For this review, take the finished solid that the model builds, in its own axes (mm). Coordinates: 2 decimals unless noted, no trailing zeros. Write each loop counter-clockwise with the first axis right and the second up, starting at its lowest first coordinate (ties: lowest second). Pieces come first, ordered by that corner, then holes.
```python
from build123d import *

# Parameters (mm, degrees)
SKETCH1_R               = 3.5
SKETCH1_R_2             = 1.05
BOSS_EXTRUDE1_DEPTH     = 60
CUT_EXTRUDE1_DEPTH      = 0.9
CUT_EXTRUDE1_DEPTH_BACK = 0.9
CUT_EXTRUDE1_START      = -30
SKETCH3_R               = 3.05
CUT_EXTRUDE2_DEPTH      = 0.9
CUT_EXTRUDE2_DEPTH_BACK = 0.9
CUT_EXTRUDE2_START      = -30
SKETCH5_W               = 7
SKETCH5_H               = 7
SKETCH5_R               = 1.05
BOSS_EXTRUDE2_DEPTH     = 60
CUT_EXTRUDE3_DEPTH      = 0.9
CUT_EXTRUDE3_DEPTH_BACK = 0.9
CUT_EXTRUDE3_START      = -30
SKETCH6_R               = 3.05
CUT_EXTRUDE4_DEPTH      = 0.9
CUT_EXTRUDE4_DEPTH_BACK = 0.9
CUT_EXTRUDE4_START      = -30
SKETCH7_W               = 8.533306348
SKETCH7_H               = 4.274424856


with BuildPart() as part:
    # Sketch1 → Boss-Extrude1 (new body)
    with BuildSketch(Plane(origin=(0, 0, 0), x_dir=(1, 0, 0), z_dir=(0, 1, 0))):
        with Locations(Location((0, 0, 0), (0, 0, 270))):
            Circle(SKETCH1_R)
        with Locations(Location((0, 0, 0), (0, 0, 270))):
            Circle(SKETCH1_R_2, mode=Mode.SUBTRACT)
    extrude(amount=BOSS_EXTRUDE1_DEPTH)

    # Sketch3 → Cut-Extrude1 (cut, two sides: drawn at the far end of the back side and taken through both)
    with BuildSketch(Plane(origin=(0, 60, 0), x_dir=(1, 0, 0), z_dir=(0, 1, 0)).offset(CUT_EXTRUDE1_START - CUT_EXTRUDE1_DEPTH_BACK)):
        with Locations(Location((0, 0, 0), (0, 0, 270))):
            Circle(SKETCH3_R)
    extrude(amount=CUT_EXTRUDE1_DEPTH + CUT_EXTRUDE1_DEPTH_BACK, mode=Mode.SUBTRACT)

    # Sketch4 → Cut-Extrude2 (cut, two sides: drawn at the far end of the back side and taken through both)
    with BuildSketch(Plane(origin=(0, 60, 0), x_dir=(1, 0, 0), z_dir=(0, 1, 0)).offset(CUT_EXTRUDE2_START - CUT_EXTRUDE2_DEPTH_BACK)):
        with BuildLine():
            Line((-4.266653174, 0), (4.266653174, 0))
            ThreePointArc((4.266653174, 0), (0, 4.266653174), (-4.266653174, 0))
        make_face()
    extrude(amount=CUT_EXTRUDE2_DEPTH + CUT_EXTRUDE2_DEPTH_BACK, mode=Mode.SUBTRACT)

    # Sketch5 → Boss-Extrude2 (add)
    with BuildSketch(Plane.XZ):
        Rectangle(SKETCH5_W, SKETCH5_H)
        with Locations(Location((0, 0, 0), (0, 0, 90))):
            Circle(SKETCH5_R, mode=Mode.SUBTRACT)
    extrude(amount=-BOSS_EXTRUDE2_DEPTH)

    # Sketch6 → Cut-Extrude3 (cut, two sides: drawn at the far end of the back side and taken through both)
    with BuildSketch(Plane(origin=(0, 60, 0), x_dir=(1, 0, 0), z_dir=(0, 1, 0)).offset(CUT_EXTRUDE3_START - CUT_EXTRUDE3_DEPTH_BACK)):
        with Locations(Location((0, 0, 0), (0, 0, 270))):
            Circle(SKETCH6_R)
    extrude(amount=CUT_EXTRUDE3_DEPTH + CUT_EXTRUDE3_DEPTH_BACK, mode=Mode.SUBTRACT)

    # Sketch7 → Cut-Extrude4 (cut, two sides: drawn at the far end of the back side and taken through both)
    with BuildSketch(Plane(origin=(0, 60, 0), x_dir=(1, 0, 0), z_dir=(0, 1, 0)).offset(CUT_EXTRUDE4_START - CUT_EXTRUDE4_DEPTH_BACK)):
        with Locations((0, 2.137212428)):
            Rectangle(SKETCH7_W, SKETCH7_H)
    extrude(amount=CUT_EXTRUDE4_DEPTH + CUT_EXTRUDE4_DEPTH_BACK, mode=Mode.SUBTRACT)


solid = part.part
```
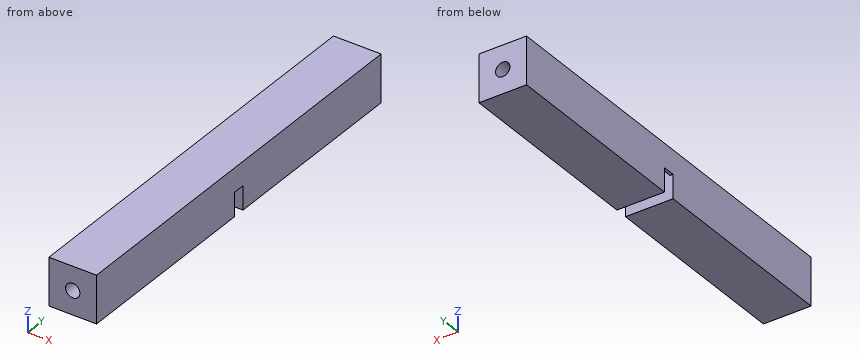
1) Consider section D-D (x = 2.5). Give the boundary of the cut face in (y, z).
2) Clearance check with flat-ended pins moving along their axes: P1, Ø1.9, axis at x = 0, z = 0, coming from the -Y side; P2, Ø3.5, axis at x = 1, z = -0.5, coming from the -Y side. State where each tip first meets the part, or that it passes through.
3) For L1, parallel to Z at x = 0, y = 22; L2, parallel to Y at x = 2.25, z = -2, list the stretches that pass through material, from the lowest coordinate up.
4) Consider section B-B (x = 0). Give the boundary of the cut face in (y, z).
5) Consider section C-C (z = 2.25). Give the boundary of the cut face in (x, y), then the cut area to 3 significant figures.
6) Consider section A-A (y = 16.5). Give the boundary of the cut face in (x, z).
Results:
1. outline: (0, -3.5) - (29.1, -3.5) - (29.1, 1.75) - (30.9, 1.75) - (30.9, -3.5) - (60, -3.5) - (60, 3.5) - (0, 3.5) - close
2. P1: passes through
2. P2: stops at y = 0
3. L1: z = -3.5 to -1.05, 1.05 to 3.5
3. L2: y = 0 to 29.1, 30.9 to 60
4. outline: (0, -3.5) - (29.1, -3.5) - (29.1, -1.05) - (0, -1.05) - close; (0, 1.05) - (29.1, 1.05) - (29.1, 3.05) - (30.9, 3.05) - (30.9, 1.05) - (60, 1.05) - (60, 3.5) - (0, 3.5) - close; (30.9, -3.5) - (60, -3.5) - (60, -1.05) - (30.9, -1.05) - close
5. outline: (-3.5, 0) - (3.5, 0) - (3.5, 60) - (-3.5, 60) - close; hole (-2.06, 29.1) - (2.06, 29.1) - (2.06, 30.9) - (-2.06, 30.9) - close
5. area: 413 mm2
6. outline: (-3.5, -3.5) - (3.5, -3.5) - (3.5, 3.5) - (-3.5, 3.5) - close; hole circle Ø2.1 at (0, 0)
